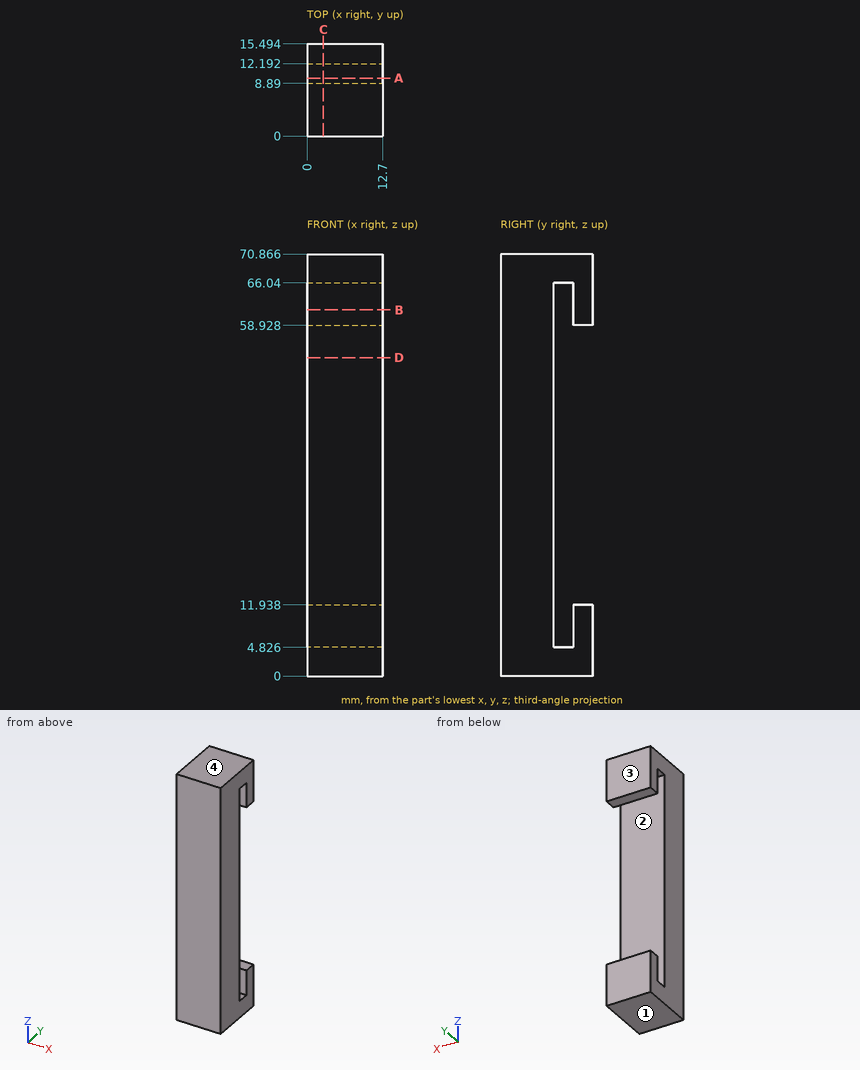
Could you check a few things on this drawing? It's one solid part, dimensions in mm from its lowest x, y, z. Coordinates: 2 decimals unless noted, no trailing zeros. Order: outer loops, then holes, each group sorted by start corner. A loop starts at its lowest first (then second) coordinate and runs counter-clockwise, first axis right, second up.
1. Thinking about a two-plate mould opening in Z: for the marked faces 1, 2, 3 and 4, which applies, +Z half, -Z half, draft (parallel to the pull), parting line (faces both ways), or undercut?
2. If we section it at C-C (x = 2.75): Please give me the cut outline in (y, z).
3. If we section it at B-B (z = 61.5): Please give me the cut outline in (x, y).
4. I'm going to push a flat-ended pin straight in: pin 1 (4 mm diameter, centred on x = 5.5, z = 30.5, fed in from +Y). Where does the tip first touch, or does it pass through?
5. If we section it at A-A (y = 9.75): Please give me the cut outline in (x, z), then the cut area to 3 significant figures.
6. I need wall thicknesses on line 1 (Z direction, x = 9, y = 14.25); line 2 (Z direction, x = 12.25, y = 12); line 3 (Y direction, x = 11.25, z = 8). Which ranges of each line are inside material? Lowest first, please.
7. If we section it at D-D (z = 53.5): Please give me the cut outline in (x, y), then the cut area to 3 significant figures.
Entries:
1. face 1: -Z half
1. face 2: undercut
1. face 3: draft
1. face 4: +Z half
2. outline: (0, 0) - (15.49, 0) - (15.49, 11.94) - (12.19, 11.94) - (12.19, 4.83) - (8.89, 4.83) - (8.89, 66.04) - (12.19, 66.04) - (12.19, 58.93) - (15.49, 58.93) - (15.49, 70.87) - (0, 70.87) - close
3. outline: (0, 0) - (12.7, 0) - (12.7, 8.89) - (0, 8.89) - close; (0, 12.19) - (12.7, 12.19) - (12.7, 15.49) - (0, 15.49) - close
4. pin 1: stops at y = 8.89
5. outline: (0, 0) - (12.7, 0) - (12.7, 4.83) - (0, 4.83) - close; (0, 66.04) - (12.7, 66.04) - (12.7, 70.87) - (0, 70.87) - close
5. area: 123 mm2
6. line 1: z = 0 to 11.94, 58.93 to 70.87
6. line 2: z = 0 to 4.83, 66.04 to 70.87
6. line 3: y = 0 to 8.89, 12.19 to 15.49
7. outline: (0, 0) - (12.7, 0) - (12.7, 8.89) - (0, 8.89) - close
7. area: 113 mm2
